Design review of the part built by this model. Coordinates are the model's own, in mm. Coordinates: 2 decimals unless noted, no trailing zeros. Order: outer loops, then holes, each group sorted by start corner. A loop starts at its lowest first (then second) coordinate and runs counter-clockwise, first axis right, second up. Notation, with made-up numbers: M 1,11.5 L 41,11.5 A8 cw 41,26.5 Z; hole C -36.75,-33 d6. An arc over 180 degrees is marked long. Answer as a JSON object with one key per item and string values.
Autodesk Inventor part; units mm, degrees
ref_plane "YZ Plane" through (0, 0, 0) normal (1, 0, 0) x (0, 1, 0)
ref_plane "XZ Plane" through (0, 0, 0) normal (0, 1, 0) x (-1, 0, 0)
ref_plane "XY Plane" through (0, 0, 0) normal (0, 0, 1) x (1, 0, 0)
sketch "Sketch1" plane through (0, 0, 0) normal (0, 1, 0) x (-1, 0, 0)
  line L0 (4, 14) -> (-86, 14)
  line L1 (-86, 14) -> (-86, -736)
  line L2 (-86, -736) -> (4, -736)
  line L3 (4, -736) -> (4, 14)
  point P0 (0, 0)
  dimension "d0" = 750
  dimension "d1" = 90
extrude "Extrusion1" add sketch "Sketch1" along normal blind 20
sketch "Sketch2" plane through (0, 20, 0) normal (0, 1, 0) x (1, 0, 0)
  line L0 (100, -14) -> (18, -14)
  line L1 (18, -14) -> (18, 66)
  line L2 (18, 66) -> (100, 66)
  line L3 (100, 66) -> (100, -14)
  line L4 (18, 66) -> (100, 228)
  line L5 (100, 228) -> (100, 66)
  line L6 (18, -14) -> (27, -14)
  line L7 (27, -14) -> (27, -14)
  line L8 (-4, -14) -> (86, -14)
  point P0 (0, 0)
  dimension "d10" = 0
  dimension "d11" = 80
  dimension "d13" = 82
  dimension "d14" = 82
  dimension "d15" = 162
  dimension "d16" = 162
  dimension "d17" = 9
  dimension "d18" = 0
  dimension "d19" = 22
  dimension "d20" = 0
extrude "Extrusion2" cut sketch "Sketch2" against normal blind 25
sketch "Sketch3" plane through (0, 20, 0) normal (0, 1, 0) x (1, 0, 0)
  line L0 (86, 736) -> (-4, 736)
  line L1 (86, 736) -> (66, 736)
  line L2 (66, 736) -> (66, -31)
  line L3 (66, -31) -> (86, -31)
  line L4 (86, -31) -> (86, 736)
  line L5 (-4, 736) -> (-4, -14)
  point P0 (0, 0)
  dimension "d7" = 70
extrude "Extrusion3" cut sketch "Sketch3" against normal blind 30
properties part number "YflanecYcrepA" material "Aluminum 6061"
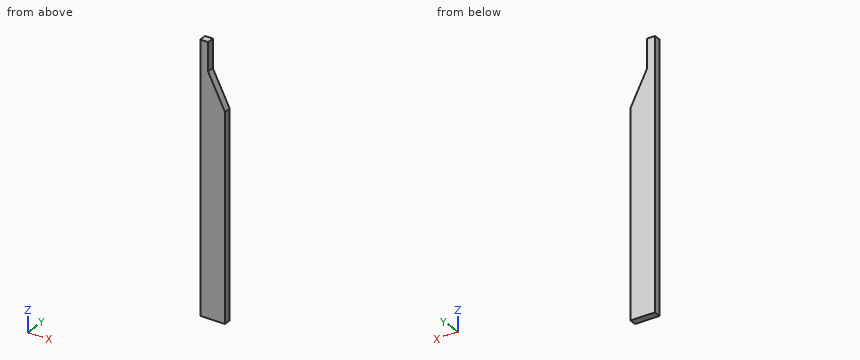
1) Add section A-A (y = 11.25). State the section outline as (x, z) points, and give its area (3 significant figures).
Taken from the geometry:
{"outline": "M -4,-736 L 66,-736 L 66,-160.83 L 18,-66 L 18,14 L -4,14 Z", "area": "46,400 mm2"}
2) Insertion check: pin 1 Ø8 at (x, y) = (55, 9) entering from +Z. The pin has a flat end and moves straight along its axis. Give the tip position at first contact, or say it passes through.
Taken from the geometry:
{"pin 1": "stops at z = -131.2"}
3) Add section B-B (x = 30). State the section outline as (y, z) points.
Taken from the geometry:
{"outline": "M 0,-736 L 20,-736 L 20,-89.71 L 0,-89.71 Z"}
4) To check wall thickness, follow L1, parallel to X at y = 1, z = -24.5; L2, parallel to X at y = 19, z = -101; L3, parallel to Z at x = 26.5, y = 2.75. State the ranges of each line that lie inside material, in increasing order.
Taken from the geometry:
{"L1": "x = -4 to 18", "L2": "x = -4 to 35.72", "L3": "z = -736 to -82.79"}
5) Add section C-C (z = -140.5). State the section outline as (x, y) points.
Taken from the geometry:
{"outline": "M -4,0 L 55.71,0 L 55.71,20 L -4,20 Z"}
